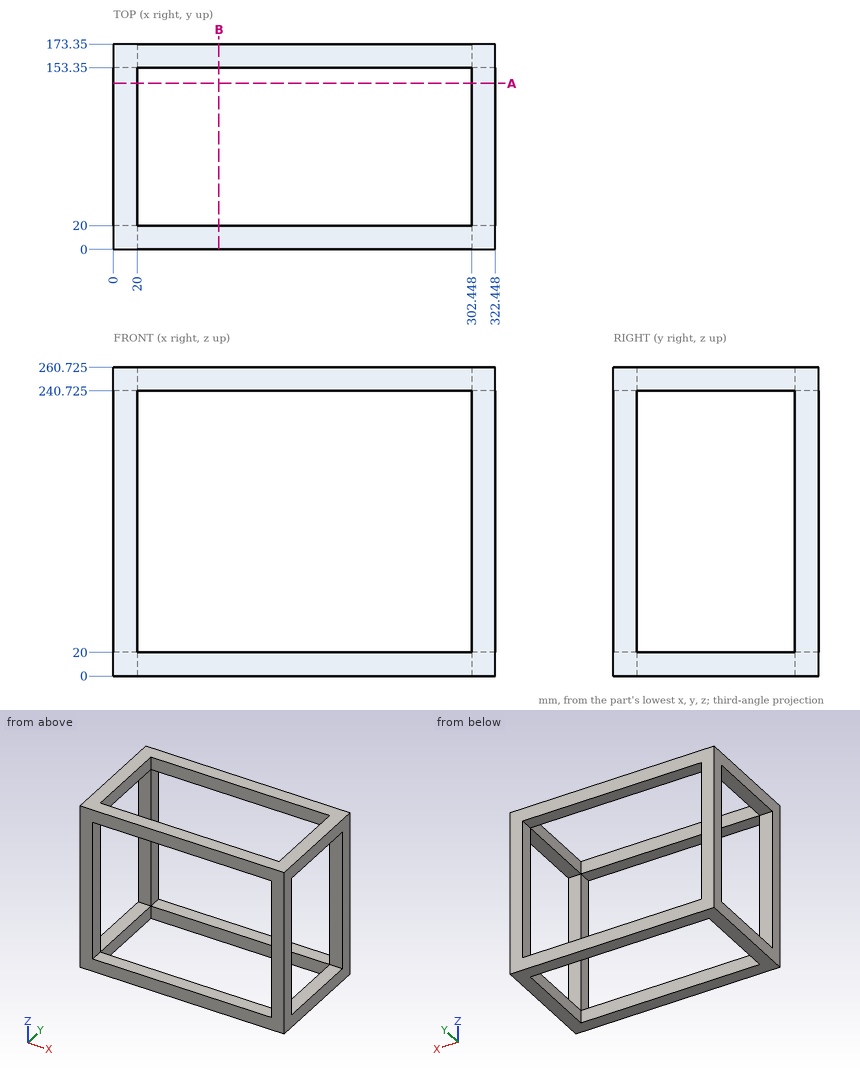
Geometry check sheet. Reference: drawing and pictorial views, mm from the part's lowest x, y, z. Round coordinates to 2 decimals unless told otherwise and drop trailing zeros. Order: outer loops, then holes, each group sorted by start corner. A loop starts at its lowest first (then second) coordinate and runs counter-clockwise, first axis right, second up. Notation, with made-up numbers: M 52,-5.5 L 58,-5.5 A26 cw 58,12.5 Z; hole C -28.75,-11 d8. An arc over 180 degrees is marked long. Answer in a Markdown table with one row per item.
(1) Sectioned sample at A-A, the plane y = 140. Record the cut outline in (x, z) (3 decimals), and give its area (3 significant figures).
Responses:
| item | result |
|---|---|
| outline | M 0,0 L 20,0 L 20,20 L 0,20 Z; M 0,240.725 L 20,240.725 L 20,260.725 L 0,260.725 Z; M 302.448,0 L 322.448,0 L 322.448,20 L 302.448,20 Z; M 302.448,240.725 L 322.448,240.725 L 322.448,260.725 L 302.448,260.725 Z |
| area | 1,600 mm² |
(2) Sectioned sample at B-B, the plane x = 89. Record the cut outline in (y, z) (3 decimals).
Responses:
| item | result |
|---|---|
| outline | M 0,0 L 20,0 L 20,20 L 0,20 Z; M 0,240.725 L 20,240.725 L 20,260.725 L 0,260.725 Z; M 153.35,0 L 173.35,0 L 173.35,20 L 153.35,20 Z; M 153.35,240.725 L 173.35,240.725 L 173.35,260.725 L 153.35,260.725 Z |
(3) Scan lines: probe 1 along Y at (x, z) = (306, 73.5); probe 2 along Z at (x, y) = (69.5, 14) (3 decimals); probe 3 along X at (y, z) = (158, 70.5). Record each from-to range of solid material in increasing order. Write a range as from..to.
Responses:
| item | result |
|---|---|
| probe 1 | y = 0..20, 153.35..173.35 |
| probe 2 | z = 0..20, 240.725..260.725 |
| probe 3 | x = 0..20, 302.45..322.45 |
